Here's the drawing with two shaded views (mm, measured from the low corner). I have some questions. A direction names the side the tool comes from. Round coordinates to 2 decimals unless told otherwise and drop trailing zeros. Order: outer loops, then holes, each group sorted by start corner. A loop starts at its lowest first (then second) coordinate and runs counter-clockwise, first axis right, second up.
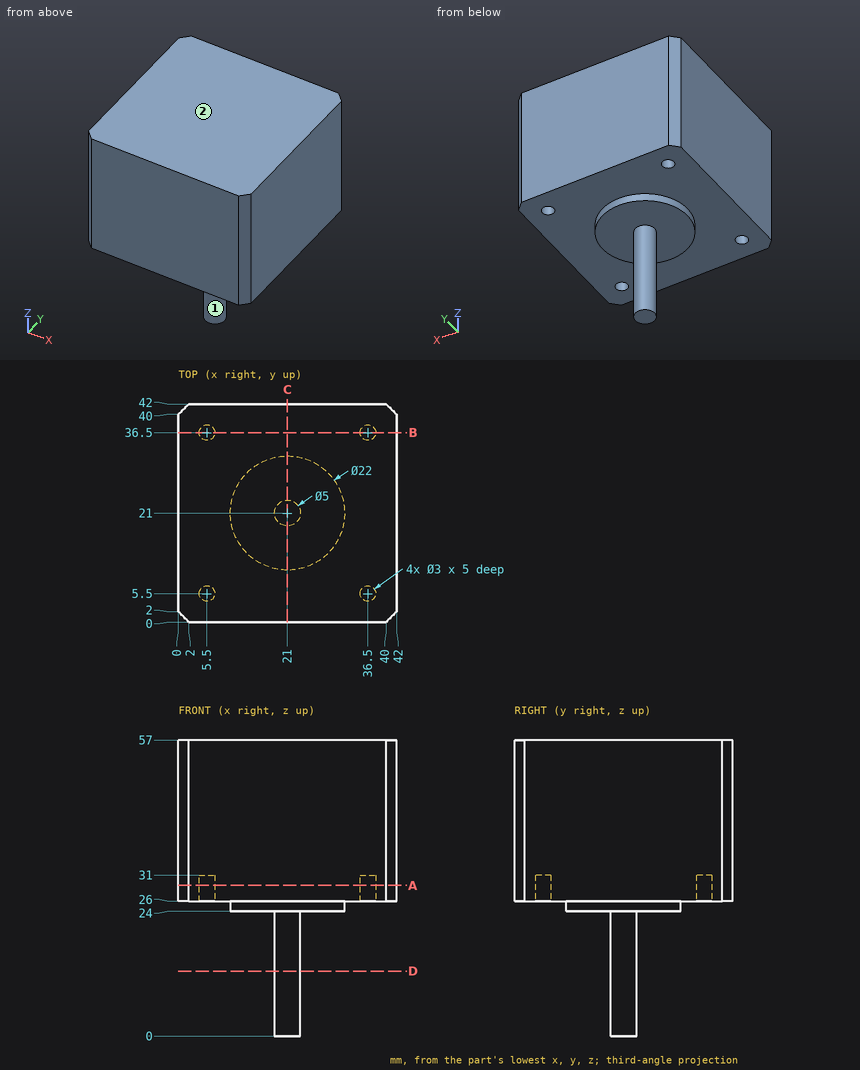
1. On a 3-axis mill with a long thin cutter (end or side, diameter ignored), from which of +Z, -Z, +X, -X, +Y, -Y can I reach the whole of each face in a straight line? I mean the marked faces 1 and 2. Say none if no direction works.
Evaluation:
face 1: -Z
face 2: +Z, +X, -X, +Y, -Y
2. If we section it at C-C, the plane x = 21: Write out the boundary of the cut face in (y, z).
Evaluation:
outline: (0, 26) - (10, 26) - (10, 24) - (18.5, 24) - (18.5, 0) - (23.5, 0) - (23.5, 24) - (32, 24) - (32, 26) - (42, 26) - (42, 57) - (0, 57) - close
3. If we section it at D-D, the plane z = 12.5: Write out the boundary of the cut face in (x, y).
Evaluation:
outline: circle Ø5 at (21, 21)
4. I'm going to push flat-ended pins straight in: P1, Ø0.9, axis at x = 37, y = 6, coming from the -Z side; P2, Ø2, axis at x = 12.5, y = 31, coming from the -Z side; P3, Ø6, axis at y = 25, z = 19, coming from the -X side. Where does each tip first touch, or does it pass through?
Evaluation:
P1: stops at z = 31
P2: stops at z = 26
P3: stops at x = 18.71
5. I need wall thicknesses on probe 1 along Y at (x, z) = (5.5, 29.6); probe 2 along Y at (x, z) = (5, 29); probe 3 along Z at (x, y) = (26, 15.5). Which ranges of each line are inside material? Lowest first, please.
Evaluation:
probe 1: y = 0 to 4, 7 to 35, 38 to 42
probe 2: y = 0 to 4.09, 6.91 to 35.09, 37.91 to 42
probe 3: z = 24 to 57
6. If we section it at A-A, the plane z = 29: Write out the boundary of the cut face in (x, y).
Evaluation:
outline: (0, 2) - (2, 0) - (40, 0) - (42, 2) - (42, 40) - (40, 42) - (2, 42) - (0, 40) - close; hole circle Ø3 at (5.5, 5.5); hole circle Ø3 at (5.5, 36.5); hole circle Ø3 at (36.5, 5.5); hole circle Ø3 at (36.5, 36.5)
7. If we section it at B-B, the plane y = 36.5: Write out the boundary of the cut face in (x, z), and give its area (3 significant figures).
Evaluation:
outline: (0, 26) - (4, 26) - (4, 31) - (7, 31) - (7, 26) - (35, 26) - (35, 31) - (38, 31) - (38, 26) - (42, 26) - (42, 57) - (0, 57) - close
area: 1,270 mm2
